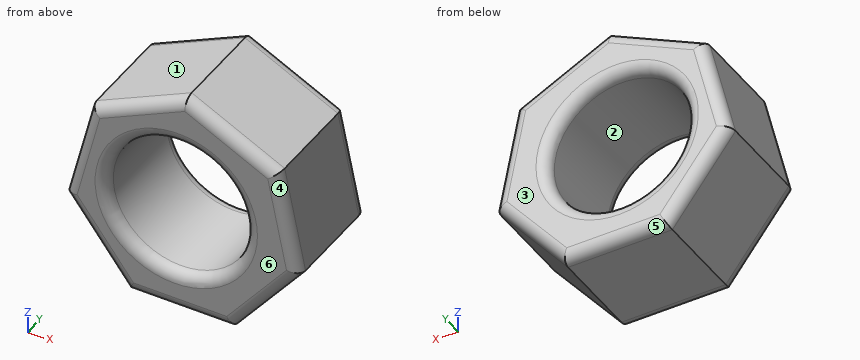
```python
from build123d import *

# Parameters (mm, degrees)
F1_DEPTH = 50
F2_R     = 30
F3_DEPTH = 50.001
F4_R     = 5


with BuildPart() as f1:
    # F0 (on Front) → F1 (new body)
    with BuildSketch(Plane.XZ):
        Polygon((43.8775578274, 31.4054595038), (3.7867815374, 51.8438952675), (-37.1888211604, 33.242820472), (-48.1937856847, -10.3907761688), (-20.9411492883, -46.1999064214), (24.0472969699, -47.2195648323), (52.8943354603, -12.6819278209), align=None)
    extrude(amount=F1_DEPTH)

    # F2 (on Front) → F3 (cut, through all)
    with BuildSketch(Plane.XZ):
        Circle(F2_R)
    extrude(amount=F3_DEPTH, mode=Mode.SUBTRACT)

    # F4
    f4_edges = [f1.edges().sort_by_distance(p)[0] for p in [
        (38.470816, -50, -29.950746),
        (1.553074, -50, -46.709736),
        (48.385947, -50, 9.361766),
        (-34.567467, -50, -28.295341),
        (23.83217, -50, 41.624677),
        (-42.691303, -50, 11.426022),
        (-16.70102, -50, 42.543358),
        (-30, -50, 0),
        (38.470816, 0, -29.950746),
        (1.553074, 0, -46.709736),
        (48.385947, 0, 9.361766),
        (-34.567467, 0, -28.295341),
        (23.83217, 0, 41.624677),
        (-42.691303, 0, 11.426022),
        (-16.70102, 0, 42.543358),
        (-30, 0, 0),
    ]]
    fillet(f4_edges, radius=F4_R)


solid = f1.part
```
Check sheet for the modelled part. Datum: model origin and axes. Units: mm. Face numbers are marked on the shaded views. A direction names the side the tool comes from. Round coordinates to 2 decimals unless told otherwise and drop trailing zeros. Write each loop counter-clockwise with the first axis right and the second up, starting at its lowest first coordinate (ties: lowest second). Pieces come first, ordered by that corner, then holes. Notation, with made-up numbers: (5, 56) -> (11, 56) arc R32 cw to (11, 83) -> close; hole circle Ø9 at (4, 64). An arc over 180 degrees is marked (long way). One line per question, with ' | ' between items. Start each with the question number.
1. Scan lines: line 1 along X through (y, z) = (-35, -16.5); line 2 along Z through (x, y) = (23.5, -19); line 3 along Z through (x, y) = (16, -35). Record each from-to range of solid material in increasing order. Write a range as from..to.
2. Release check for a two-part mould opening along X. For the marked faces 1, 2, 3 and 4 record: +X half, -X half, draft (parallel to the pull), parting line (faces both ways), or undercut.
3. Sectioned sample at A-A, the plane y = -26.5. Record the cut outline in (x, z).
4. Depth check by flat-ended pin: pin 1 (12 mm diameter, centred on x = -7, y = -39, fed in from +Z); pin 2 (4 mm diameter, centred on x = -28.5, y = -29.5, fed in from -Z); pin 3 (12 mm diameter, centred on x = -5.5, y = -13.5, fed in from -Z). Enter the tip coordinate at first touch or a pass-through.
5. Set-up check for the marked faces 5 and 6: record each of +Z, -Z, +X, -X, +Y, -Y from which the full face is reachable in a straight line by a thin tool's end or side.
Taken from the geometry:
1) line 1: x = -43.54..-25.05, 25.05..49.71 | line 2: z = -47.21..-18.65, 18.65..41.79 | line 3: z = -47.04..-25.38, 25.38..45.62
2) face 1: -X half | face 2: undercut | face 3: draft | face 4: +X half
3) outline: (-48.19, -10.39) -> (-20.94, -46.2) -> (24.05, -47.22) -> (52.89, -12.68) -> (43.88, 31.41) -> (3.79, 51.84) -> (-37.19, 33.24) -> close; hole circle Ø60 at (0, 0)
4) pin 1: stops at z = 49.67 | pin 2: stops at z = -38.9 | pin 3: stops at z = -46.69
5) face 5: -Z, -X, +Y | face 6: +Z, -Z, +X, -X, -Y
